from build123d import *

# Parameters (mm, degrees)
BOSS_EXTRUDE1_DEPTH           = 1.6
SKETCH4_R                     = 2.3
BOSS_EXTRUDE2_DEPTH           = 2
M2_CLEARANCE_HOLE1_AT_2_COUNT = 2
M2_CLEARANCE_HOLE1_AT_2_PITCH = 12.5
M2_CLEARANCE_HOLE1_AT_3_COUNT = 2
M2_CLEARANCE_HOLE1_AT_3_PITCH = 24.43869882
M2_CLEARANCE_HOLE1_AT_4_COUNT = 2
M2_CLEARANCE_HOLE1_AT_4_PITCH = 21
CHAMFER1_SIZE                 = 2
CHAMFER1_SIZE_2               = 0.8


with BuildPart() as part:
    # Sketch1 → Boss-Extrude1 (new body)
    with BuildSketch(Plane.XY):
        with BuildLine():
            Line((10.50000068, 13.480003898), (-10.50000068, 13.480003898))
            ThreePointArc((-10.50000068, 13.480003898), (-12.621321024, 12.601324241), (-13.50000068, 10.480003898))
            Line((-13.50000068, 10.480003898), (-13.50000068, -7.519996102))
            ThreePointArc((-13.50000068, -7.519996102), (-12.621321024, -9.641316446), (-10.50000068, -10.519996102))
            Line((-10.50000068, -10.519996102), (10.50000068, -10.519996102))
            ThreePointArc((10.50000068, -10.519996102), (12.621321024, -9.641316446), (13.50000068, -7.519996102))
            Line((13.50000068, -7.519996102), (13.50000068, 10.480003898))
            ThreePointArc((13.50000068, 10.480003898), (12.621321024, 12.601324241), (10.50000068, 13.480003898))
        make_face()
    extrude(amount=BOSS_EXTRUDE1_DEPTH)

    # Sketch4 → Boss-Extrude2 (add)
    with BuildSketch(Plane(origin=(0, 0, 0), x_dir=(-1, 0, 0), z_dir=(0, 0, -1))):
        with Locations((-10.500001265, 4.980003898)):
            Circle(SKETCH4_R)
        with Locations((10.499998735, 4.98000488)):
            Circle(SKETCH4_R)
        with Locations((10.50000068, -7.519996102)):
            Circle(SKETCH4_R)
        with Locations((-10.50000068, -7.519996102)):
            Circle(SKETCH4_R)
    extrude(amount=BOSS_EXTRUDE2_DEPTH)

    # Sketch3 → M2 Clearance Hole1 (revolve, cut)
    with BuildSketch(Plane(origin=(10.500001265, 4.980003898, 1.6), x_dir=(0, -1, 0), z_dir=(1, 0, 0))):
        Polygon((0, 0), (0, 3.6), (1.1, 3.6), (1.1, 0.965685425), (1.5, 0), align=None)
    m2_clearance_hole1 = revolve(axis=Axis((10.500001265, 4.980003898, 7.95), (0, 0, -1)), mode=Mode.SUBTRACT)

    # M2 Clearance Hole1 at 2: M2 Clearance Hole1 ×2
    with Locations(*[(0, -i * M2_CLEARANCE_HOLE1_AT_2_PITCH, 0) for i in range(1, M2_CLEARANCE_HOLE1_AT_2_COUNT)]):
        add(m2_clearance_hole1, mode=Mode.SUBTRACT)

    # M2 Clearance Hole1 at 3: M2 Clearance Hole1 ×2
    with Locations(*[Vector(-0.8592929083374752, -0.5114838195690296, 0) * (i * M2_CLEARANCE_HOLE1_AT_3_PITCH) for i in range(1, M2_CLEARANCE_HOLE1_AT_3_COUNT)]):
        add(m2_clearance_hole1, mode=Mode.SUBTRACT)

    # M2 Clearance Hole1 at 4: M2 Clearance Hole1 ×2
    with Locations(*[(-i * M2_CLEARANCE_HOLE1_AT_4_PITCH, 0, 0) for i in range(1, M2_CLEARANCE_HOLE1_AT_4_COUNT)]):
        add(m2_clearance_hole1, mode=Mode.SUBTRACT)

    # Chamfer1
    # the kernel refuses this chamfer: 2, 0.8 mm, written as the material it takes off along each edge
    with BuildSketch(Plane(origin=(10.500001265, 4.980003898, -2), x_dir=(-1, 0, 0), z_dir=(0, -1, 0))) as chamfer1_piece_1_section:
        Polygon((2.3, -CHAMFER1_SIZE), (2.3 - CHAMFER1_SIZE_2, 0), (2.3, 0), align=None)
    chamfer1_piece_1 = revolve(axis=Axis((10.500001265, 4.980003898, -2), (0, 0, -1)), mode=Mode.PRIVATE)
    chamfer1_piece_1 = split(chamfer1_piece_1, bisect_by=Plane(origin=(12.406400558, 4.980003898, 0), z_dir=(0, 0, -1)), keep=Keep.TOP, mode=Mode.PRIVATE)
    add(chamfer1_piece_1, mode=Mode.SUBTRACT)
    with BuildSketch(Plane(origin=(-10.499998735, 4.98000488, -2), x_dir=(-1, 0, 0), z_dir=(0, -1, 0))) as chamfer1_piece_2_section:
        Polygon((2.3, -CHAMFER1_SIZE), (2.3 - CHAMFER1_SIZE_2, 0), (2.3, 0), align=None)
    chamfer1_piece_2 = revolve(axis=Axis((-10.499998735, 4.98000488, -2), (0, 0, -1)), mode=Mode.PRIVATE)
    chamfer1_piece_2 = split(chamfer1_piece_2, bisect_by=Plane(origin=(-8.593599442, 4.98000488, 0), z_dir=(0, 0, -1)), keep=Keep.TOP, mode=Mode.PRIVATE)
    add(chamfer1_piece_2, mode=Mode.SUBTRACT)
    with BuildSketch(Plane(origin=(-10.50000068, -7.519996102, -2), x_dir=(-1, 0, 0), z_dir=(0, -1, 0))) as chamfer1_piece_3_section:
        Polygon((2.3, -CHAMFER1_SIZE), (2.3 - CHAMFER1_SIZE_2, 0), (2.3, 0), align=None)
    chamfer1_piece_3 = revolve(axis=Axis((-10.50000068, -7.519996102, -2), (0, 0, -1)), mode=Mode.PRIVATE)
    chamfer1_piece_3 = split(chamfer1_piece_3, bisect_by=Plane(origin=(-8.593601387, -7.519996102, 0), z_dir=(0, 0, -1)), keep=Keep.TOP, mode=Mode.PRIVATE)
    add(chamfer1_piece_3, mode=Mode.SUBTRACT)
    with BuildSketch(Plane(origin=(10.50000068, -7.519996102, -2), x_dir=(-1, 0, 0), z_dir=(0, -1, 0))) as chamfer1_piece_4_section:
        Polygon((2.3, -CHAMFER1_SIZE), (2.3 - CHAMFER1_SIZE_2, 0), (2.3, 0), align=None)
    chamfer1_piece_4 = revolve(axis=Axis((10.50000068, -7.519996102, -2), (0, 0, -1)), mode=Mode.PRIVATE)
    chamfer1_piece_4 = split(chamfer1_piece_4, bisect_by=Plane(origin=(12.406399973, -7.519996102, 0), z_dir=(0, 0, -1)), keep=Keep.TOP, mode=Mode.PRIVATE)
    add(chamfer1_piece_4, mode=Mode.SUBTRACT)


solid = part.part
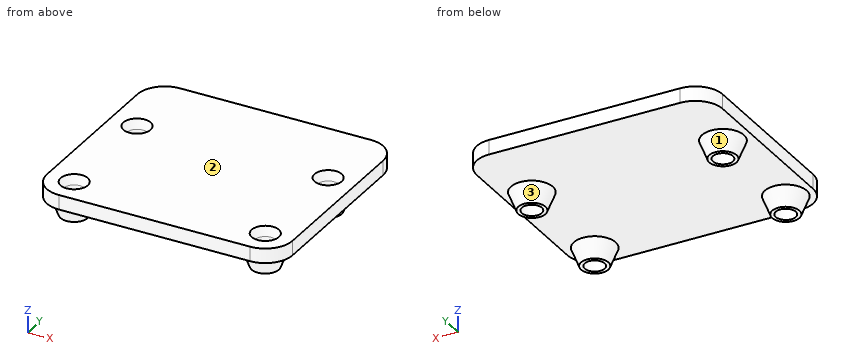
Build history of the part. All positions in model axes, mm. Face numbers are marked on the shaded views. Coordinates: 2 decimals unless noted, no trailing zeros. Order: outer loops, then holes, each group sorted by start corner. A loop starts at its lowest first (then second) coordinate and runs counter-clockwise, first axis right, second up. Notation, with made-up numbers: (81, 46) - (134, 46) arc R23 ccw to (134, 71) - close; hole circle Ø11 at (-2.5, -21). An arc over 180 degrees is marked (long way). Write item = value, one per line. Start each with the question number.
1) Saw through at A-A on x = -2. Write the cut outline in (y, z), then the cut area to 3 significant figures.
2) Saw through at B-B on y = 4.5. Count the separate pieces of the cut face and the enclosed holes in it, then the cut area to 3 significant figures.
3) Wall check: line 1 along Y through (x, z) = (11.25, 1.15); line 2 along X through (y, z) = (-8.5, -0.7); line 3 along Z through (x, y) = (-0.25, -4.5). Give the ranges that are in metal, low to high. Write a range as from..to.
4) Flat gauge pins, fed straight in: pin 1 Ø2.5 at (x, y) = (-10.5, -7.52) entering from +Z; pin 2 Ø1 at (x, y) = (4.5, 7.5) entering from -Z. Where does each tip first touch, or does it go through?
5) Saw through at D-D on y = -1.25. Write the cut outline in (x, z), then the cut area to 3 significant figures.
6) Two-plate mould, pull along X, no slides. Class the marked faces 1, 2 and 3: pulls with the +X half, pulls with the -X half, needs draft (parallel to the pull), parting line crosses it, or undercut.
From the geometry:
q1.outline = (-10.52, 0) - (13.48, 0) - (13.48, 1.6) - (-10.52, 1.6) - close
q1.area = 38.4 mm^2
q2.separate_pieces = 3
q2.enclosed_holes = 0
q2.area = 42.8 mm^2
q3.line_1 = -10.42..-8.6, -6.44..3.9, 6.06..13.38
q3.line_2 = -12.27..-11, -10..-8.73, 8.73..10, 11..12.27
q3.line_3 = 0..1.6
q4.pin_1 = 1
q4.pin_2 = 0
q5.outline = (-13.5, 0) - (13.5, 0) - (13.5, 1.6) - (-13.5, 1.6) - close
q5.area = 43.2 mm^2
q6.face_1 = undercut
q6.face_2 = needs draft
q6.face_3 = undercut
